The drawing under review shows one solid part. Ordinate dimensions are in mm from its lowest x, y, z. A direction names the side the tool comes from. Give positions to 0.01 mm unless a question says otherwise; leave off trailing zeros. Order: outer loops, then holes, each group sorted by start corner. A loop starts at its lowest first (then second) coordinate and runs counter-clockwise, first axis right, second up. Notation, with made-up numbers: (18, -14) - (48, -14) arc R23 cw to (48, -1) - close; hole circle Ø10 at (8, -24.75). An arc over 180 degrees is marked (long way). Write item = value, one per line. Start each with the question number.
1. Mouldability with a two-part tool opening along Z and no side actions: class the marked faces 1, 2 and 3 as pulls with the +Z half, pulls with the -Z half, needs draft (parallel to the pull), parting line crosses it, or undercut.
2. We need section A-A, the plane z = 7.5. Give the boundary of the cut face in (x, y).
3. We need section D-D, the plane y = 1.25. Give the boundary of the cut face in (x, z).
4. Machinability: for the marked faces 4 and 5, which of the approach directions +Z, -Z, +X, -X, +Y, -Y give a long, thin tool a straight path to every point of the face, cutting with its end or side? Answer none if there is none.
5. We need section C-C, the plane x = 8.25. Give the boundary of the cut face in (y, z).
6. For P1, Ø6, axis at x = 13.5, y = 9, coming from the +Z side; P2, Ø5, axis at y = 9.5, z = 6.5, coming from the +X side; P3, Ø1, axis at y = 3, z = 6, coming from the +X side, all flat-tipped, find the tip position at first contact; note any pin that passes through.
7. Wall thickness on probe 1 along Y at (x, z) = (3.25, 3.25); probe 2 along X at (y, z) = (9, 7.5); probe 3 along Z at (x, y) = (7, 15.25): over which ranges is each line inside the solid? List them lowest first.
8. We need section B-B, the plane y = 11.25. Give the boundary of the cut face in (x, z), and give its area (3 significant figures).
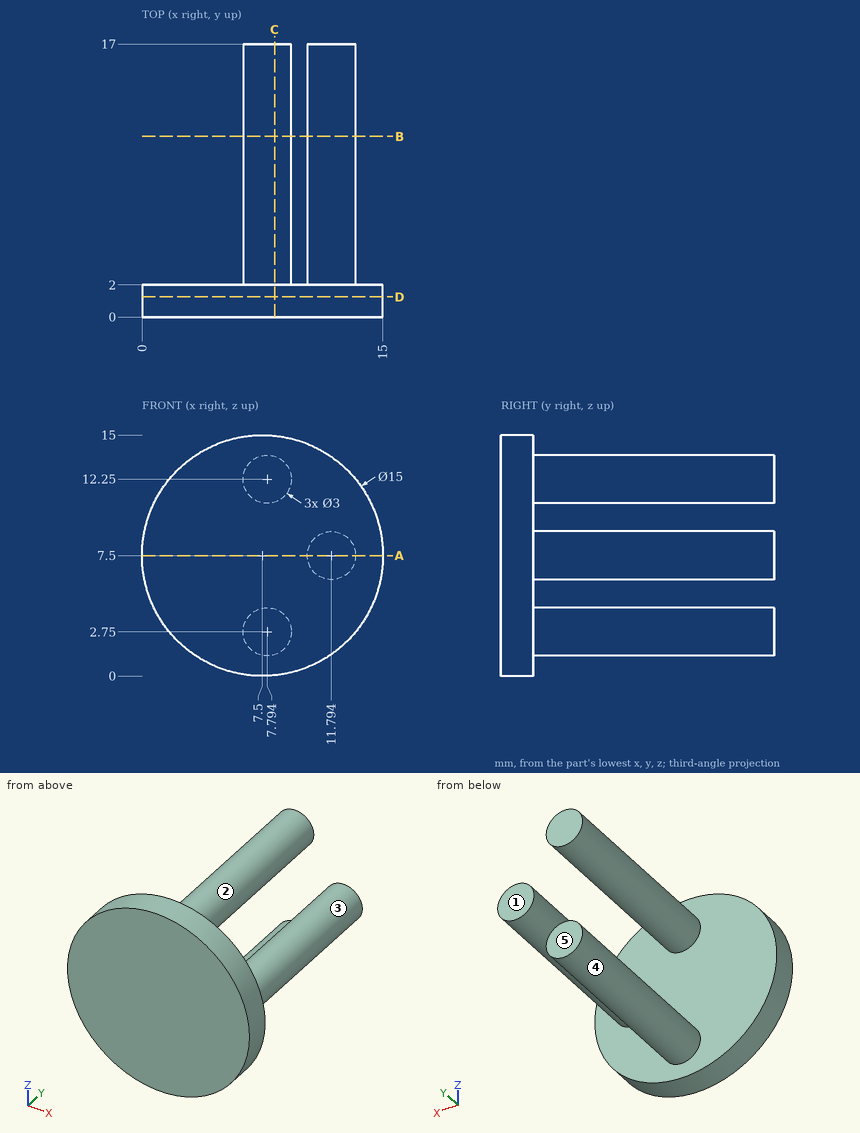
Model answer:
q1.face_1 = needs draft
q1.face_2 = undercut
q1.face_3 = parting line crosses it
q2.outline = (0, 0) - (15, 0) - (15, 2) - (13.29, 2) - (13.29, 17) - (10.29, 17) - (10.29, 2) - (0, 2) - close
q3.outline = circle Ø15 at (7.5, 7.5)
q4.face_4 = +Y
q4.face_5 = +Z, -Z, +X, -X, +Y
q5.outline = (0, 0.04) - (2, 0.04) - (2, 1.32) - (17, 1.32) - (17, 4.18) - (2, 4.18) - (2, 10.82) - (17, 10.82) - (17, 13.68) - (2, 13.68) - (2, 14.96) - (0, 14.96) - close
q6.P1 = 9
q6.P2 = 13.29
q6.P3 = 12.91
q7.probe_1 = 0 to 2
q7.probe_2 = 10.29 to 13.29
q7.probe_3 = 1.48 to 4.02, 10.98 to 13.52
q8.outline = circle Ø3 at (7.79, 2.75); circle Ø3 at (7.79, 12.25); circle Ø3 at (11.79, 7.5)
q8.area = 21.2 mm2
